Here's how the part is built. I have some questions about the finished solid (model axes, mm). Coordinates: 2 decimals unless noted, no trailing zeros. Loops run counter-clockwise (first coordinate to the right, second up) from the corner with the lowest first, then second, coordinate; pieces in that order, holes last. Notation, with made-up numbers: (-14, 13) -> (23, 13) arc R33 cw to (23, 50) -> close; hole circle Ø5 at (49.5, 12.5). An arc over 180 degrees is marked (long way). Answer as a JSON object with one key per item and string values. Group by question number.
Q1. I need wall thicknesses on line 1 (Z direction, x = 0.25, y = 26.5); line 2 (X direction, y = 37.5, z = 1.25); line 3 (Y direction, x = 3.25, z = 1.25). Which ranges of each line are inside material? Lowest first, please.
Q2. I want a section at C-C on z = -2.75. Write out the boundary of the cut face in (x, y), then the cut area to 3 significant figures.
Q3. I want a section at A-A on y = 14.5. Write out the boundary of the cut face in (x, z), then the cut area to 3 significant figures.
Q4. I'm going to push flat-ended pins straight in: pin 1 (2.5 mm diameter, centred on x = -1.5, z = 1, fed in from -Y); pin 2 (1 mm diameter, centred on x = -1.5, y = 26.5, fed in from -Z); pin 3 (1.1 mm diameter, centred on x = -1, z = 0, fed in from +Y); pin 4 (4 mm diameter, centred on x = 3, z = 2, fed in from +Y). Where does each tip first touch, or does it pass through?
Q5. Thinking about a two-plate mould opening in X: for faces 1 (the flat face through (0, 37, 0)), 2 (the cylindrical face through (-2, 18, 0)), 3 (the flat face through (-1, 37, -2)), which applies, released by +X, released by -X, zero draft, split by the parting line, or undercut?
Q6. I want a section at B-B on x = -3.25. Write out the boundary of the cut face in (y, z), then the cut area to 3 significant figures.
```python
from build123d import *

# Parameters (mm, degrees)
SKETCH1_R           = 2
BOSS_EXTRUDE1_DEPTH = 37
SKETCH2_R           = 4
BOSS_EXTRUDE2_DEPTH = 2
DOME1_FACE_RADIUS   = 4
DOME1_HEIGHT        = 1
CUT_EXTRUDE1_DEPTH  = 3
CUT_EXTRUDE1_TAPER  = 3


with BuildPart() as part:
    # Sketch1 → Boss-Extrude1 (new body)
    with BuildSketch(Plane(origin=(0, 0, 0), x_dir=(1, 0, 0), z_dir=(0, 1, 0))):
        with Locations(Location((0, 0, 0), (0, 0, 270))):
            Circle(SKETCH1_R)
    extrude(amount=BOSS_EXTRUDE1_DEPTH)

    # Sketch2 → Boss-Extrude2 (add)
    with BuildSketch(Plane(origin=(0, 37, 0), x_dir=(1, 0, 0), z_dir=(0, 1, 0))):
        with Locations(Location((0, 0, 0), (0, 0, 270))):
            Circle(SKETCH2_R)
    extrude(amount=BOSS_EXTRUDE2_DEPTH)

    # Dome1: a dome of height H over a round flat face of radius A is a cap of a sphere of radius (A * A + H * H) / (2 * H)
    dome1_r = (DOME1_FACE_RADIUS * DOME1_FACE_RADIUS + DOME1_HEIGHT * DOME1_HEIGHT) / (2 * DOME1_HEIGHT)
    dome1_base = Plane((0, 39, 0), z_dir=(0, 1, 0))
    with Locations(dome1_base.offset(DOME1_HEIGHT - dome1_r)):
        dome1_ball = Sphere(dome1_r, mode=Mode.PRIVATE)
    add(split(dome1_ball, bisect_by=dome1_base, keep=Keep.TOP, mode=Mode.PRIVATE))

    # Sketch4 → Cut-Extrude1 (cut)
    with BuildSketch(Plane(origin=(0, 40, 0), x_dir=(-1, 0, 0), z_dir=(0, -1, 0))):
        Polygon((-0.5, 0.5), (-2, 0.5), (-2, -0.5), (-0.5, -0.5), (-0.5, -2), (0.5, -2), (0.5, -0.5), (2, -0.5), (2, 0.5), (0.5, 0.5), (0.5, 2), (-0.5, 2), align=None)
    extrude(amount=CUT_EXTRUDE1_DEPTH, taper=CUT_EXTRUDE1_TAPER, mode=Mode.SUBTRACT)


solid = part.part
```
Result set:
{
 "1": {"line 1": "z = -1.98 to 1.98", "line 2": "x = -3.8 to -0.37, 0.37 to 3.8", "line 3": "y = 37 to 39.25"},
 "2": {"outline": "(-2.9, 37) -> (2.9, 37) -> (2.9, 39) arc R8.04 ccw to (-2.9, 39) -> close", "area": "13.7 mm²"},
 "3": {"outline": "circle Ø4 at (0, 0)", "area": "12.6 mm²"},
 "4": {"pin 1": "stops at y = 0", "pin 2": "stops at z = -1.73", "pin 3": "stops at y = 39.95", "pin 4": "stops at y = 39.85"},
 "5": {"face 1": "undercut", "face 2": "split by the parting line", "face 3": "zero draft"},
 "6": {"outline": "(37, -2.33) -> (39, -2.33) arc R7.85 ccw to (39, 2.33) -> (37, 2.33) -> close", "area": "10.4 mm²"}
}
